Verification items for the finished model (mm, model axes). A direction names the side the tool comes from. Give positions to 0.01 mm unless a question says otherwise; leave off trailing zeros. Loops run counter-clockwise (first coordinate to the right, second up) from the corner with the lowest first, then second, coordinate; pieces in that order, holes last. Notation, with made-up numbers: (89.5, -13.5) - (131.5, -13.5) arc R31 ccw to (131.5, 19.5) - close; hole circle Ø6 at (55, 18.5). An arc over 180 degrees is marked (long way). Put each result on its own line as item: value. Start each with the question number.
Solid Edge part; units mm, degrees
sketch "Sketch1" plane through (0, 0, 0) normal (0, 0, 1) x (1, 0, 0)
  line L0 (53.5, -43.85) -> (53.5, 43.85)
  line L1 (53.5, 43.85) -> (-53.5, 43.85)
  line L2 (-53.5, 43.85) -> (-53.5, -43.85)
  line L3 (-53.5, -43.85) -> (53.5, -43.85)
extrude "Protrusion1" add sketch "Sketch1" along normal blind 15
sketch "Sketch2" plane through (0, -43.85, 7.5) normal (0, -1, 0) x (1, 0, 0)
  line L0 (7.5, -2.5) -> (-7.5, -2.5)
  line L1 (-7.5, -2.5) -> (-7.5, -12.5)
  line L2 (-7.5, -12.5) -> (7.5, -12.5)
  line L3 (7.5, -12.5) -> (7.5, -2.5)
extrude "Corte_1" cut sketch "Sketch2" against normal blind 19
sketch "Sketch3" plane through (53.5, 0, 7.5) normal (1, 0, 0) x (0, 1, 0)
  line L0 (12.5, -2.5) -> (-12.5, -2.5)
  line L1 (-12.5, -2.5) -> (-12.5, -12.5)
  line L2 (-12.5, -12.5) -> (12.5, -12.5)
  line L3 (12.5, -12.5) -> (12.5, -2.5)
extrude "Corte_2" cut sketch "Sketch3" against normal blind 125.4573
sketch "Sketch4" plane through (0, 0, 15) normal (0, 0, 1) x (1, 0, 0)
  line L0 (51.1, -41.5) -> (51.1, 41.5)
  line L1 (51.1, 41.5) -> (-51.1, 41.5)
  line L2 (-51.1, 41.5) -> (-51.1, -41.5)
  line L3 (-51.1, -41.5) -> (51.1, -41.5)
extrude "Corte_3" cut sketch "Sketch4" against normal blind 8
sketch "Sketch5" plane through (0, 0, 7) normal (0, 0, 1) x (1, 0, 0)
  circle A0 centre (-42.5, -25) radius 2.2
  circle A1 centre (42.5, 25) radius 2.2
extrude "ProtrusiónExtruida_2" add sketch "Sketch5" along normal blind 7
sketch "Sketch6" plane through (0, 0, 7) normal (0, 0, 1) x (1, 0, 0)
  line L0 (7.5, -41.5) -> (7.5, -24.85)
  line L1 (7.5, -24.85) -> (6, -24.85)
  line L2 (6, -24.85) -> (6, -41.5)
  line L3 (6, -41.5) -> (7.5, -41.5)
  line L4 (-6, -24.85) -> (-6, -41.5)
  line L5 (-6, -41.5) -> (-7.5, -41.5)
  line L6 (-7.5, -41.5) -> (-7.5, -24.85)
  line L7 (-7.5, -24.85) -> (-6, -24.85)
extrude "Corte_4" cut sketch "Sketch6" against normal blind 21
sketch "Sketch7" plane through (0, 0, 7) normal (0, 0, 1) x (1, 0, 0)
  line L0 (-51.1, 12.5) -> (-21.1, 12.5)
  line L1 (-21.1, 12.5) -> (-21.1, 9.5)
  line L2 (-21.1, 9.5) -> (-51.1, 9.5)
  line L3 (-51.1, 9.5) -> (-51.1, 12.5)
  line L4 (51.1, 12.5) -> (21.1, 12.5)
  line L5 (21.1, 12.5) -> (21.1, 9.5)
  line L6 (21.1, 9.5) -> (51.1, 9.5)
  line L7 (51.1, 9.5) -> (51.1, 12.5)
extrude "Corte_5" cut sketch "Sketch7" against normal blind 84
sketch "Sketch8" plane through (-42.5, -25, 14) normal (0, 0, 1) x (1, 0, 0)
  circle A0 centre (0, 0) radius 1.2
  circle A1 centre (85, 50) radius 1.2
extrude "Corte_6" cut sketch "Sketch8" against normal blind 5.5
properties part number "Natanael Alc" material "PVC"
1) Section check B-B, the plane x = -1. Enter the section's corners in (y, z).
2) Scan lines: line 1 along Y through (x, z) = (-42.5, 10.05); line 2 along Y through (x, z) = (42.5, 11.35); line 3 along Y through (x, z) = (18, 13). Record each from-to range of solid material in increasing order. Write a range as from..to.
3) Section check C-C, the plane y = 25. Enter the section's corners in (x, z), plus the area to 3 significant figures.
4) Depth check by flat-ended pin: P1, Ø2, axis at x = -14.5, y = -8, coming from the +Z side; P2, Ø5, axis at x = -42, y = -24.5, coming from the +Z side; P3, Ø10, axis at x = 34.5, y = 2.5, coming from the -Z side. Enter the tip coordinate at first touch or a pass-through.
5) Section check A-A, the plane x = -42.5. Enter the section's corners in (y, z).
6) Set-up check for faces 4 (the face through (-1, -24, 0)), 5 (the face through (-4, -42, 15)), 6 (the face through (40.754, 26.339, 10.451)), 7 (the face through (0, -34, 5)), 8 (the face through (1, 0, 5)): record each of +Z, -Z, +X, -X, +Y, -Y from which the full face is reachable in a straight line by a thin tool's end or side.
7) Draft check along X on faces 1 (the face through (1, -12.5, 3)), 2 (the face through (53.5, -1, 7)), 3 (the face through (0, -24.85, 3)). Enter one of: pulls with the +X half, pulls with the -X half, needs draft (parallel to the pull), parting line crosses it, or undercut.
Results are:
1. outline: (-43.85, 5) - (-24.85, 5) - (-24.85, 0) - (-12.5, 0) - (-12.5, 5) - (12.5, 5) - (12.5, 0) - (43.85, 0) - (43.85, 15) - (41.5, 15) - (41.5, 7) - (-41.5, 7) - (-41.5, 15) - (-43.85, 15) - close
2. line 1: y = -43.85..-41.5, -27.2..-26.2, -23.8..-22.8, 41.5..43.85
2. line 2: y = -43.85..-41.5, 22.8..23.8, 26.2..27.2, 41.5..43.85
2. line 3: y = -43.85..-41.5, 41.5..43.85
3. outline: (-53.5, 0) - (53.5, 0) - (53.5, 15) - (51.1, 15) - (51.1, 7) - (44.7, 7) - (44.7, 14) - (43.7, 14) - (43.7, 8.5) - (41.3, 8.5) - (41.3, 14) - (40.3, 14) - (40.3, 7) - (-51.1, 7) - (-51.1, 15) - (-53.5, 15) - close
3. area: 805 mm2
4. P1: stops at z = 7
4. P2: stops at z = 14
4. P3: stops at z = 5
5. outline: (-43.85, 0) - (-12.5, 0) - (-12.5, 5) - (9.5, 5) - (9.5, 7) - (-22.8, 7) - (-22.8, 14) - (-23.8, 14) - (-23.8, 8.5) - (-26.2, 8.5) - (-26.2, 14) - (-27.2, 14) - (-27.2, 7) - (-41.5, 7) - (-41.5, 15) - (-43.85, 15) - close; (12.5, 0) - (43.85, 0) - (43.85, 15) - (41.5, 15) - (41.5, 7) - (12.5, 7) - close
6. face 4: -Z, +X, -X, +Y, -Y
6. face 5: +Z, +X, -X, +Y, -Y
6. face 6: +Z
6. face 7: -Z, -Y
6. face 8: -Z, +X, -X
7. face 1: needs draft
7. face 2: pulls with the +X half
7. face 3: undercut
